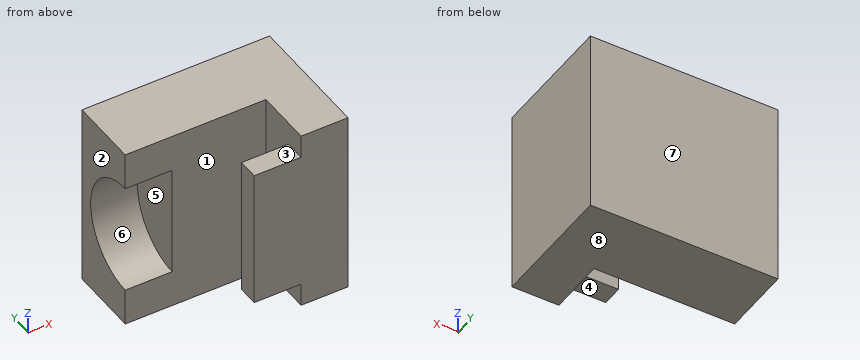
from build123d import *

# Parameters (mm, degrees)
SKETCH1_W           = 25.4
SKETCH1_H           = 9.525
BOSS_EXTRUDE1_DEPTH = 25.4
SKETCH2_W           = 6.35
SKETCH2_H           = 25.4
BOSS_EXTRUDE2_DEPTH = 7.747
SKETCH3_W           = 19.05
SKETCH3_H           = 2.794
BOSS_EXTRUDE3_DEPTH = 6.35
CUT_EXTRUDE1_DEPTH  = 6.35


with BuildPart() as part:
    # Sketch1 → Boss-Extrude1 (new body)
    with BuildSketch(Plane(origin=(0, 0, 0), x_dir=(0, 0, -1), z_dir=(1, 0, 0))):
        Rectangle(SKETCH1_W, SKETCH1_H)
    extrude(amount=BOSS_EXTRUDE1_DEPTH)

    # Sketch2 → Boss-Extrude2 (add)
    with BuildSketch(Plane.XZ.offset(4.7625)):
        with Locations((22.225, 0)):
            Rectangle(SKETCH2_W, SKETCH2_H)
    extrude(amount=BOSS_EXTRUDE2_DEPTH)

    # Sketch3 → Boss-Extrude3 (add)
    with BuildSketch(Plane.ZY.offset(-19.05)):
        with Locations((0, -11.1125)):
            Rectangle(SKETCH3_W, SKETCH3_H)
    extrude(amount=BOSS_EXTRUDE3_DEPTH)

    # Sketch4 → Cut-Extrude1 (cut)
    with BuildSketch(Plane.ZY):
        with BuildLine():
            Line((-7.62, -4.7625), (7.62, -4.7625))
            ThreePointArc((7.62, -4.7625), (0, 2.8575), (-7.62, -4.7625))
        make_face()
    extrude(amount=-CUT_EXTRUDE1_DEPTH, mode=Mode.SUBTRACT)


solid = part.part
The listing builds one solid part. Answer for the finished solid, in the listing's coordinates (mm). Face numbers are marked on the shaded views. A direction names the side the tool comes from. Coordinates: 2 decimals unless noted, no trailing zeros. Loops run counter-clockwise (first coordinate to the right, second up) from the corner with the lowest first, then second, coordinate; pieces in that order, holes last. Notation, with made-up numbers: (-9, -13) -> (18, -13) arc R35 cw to (18, 22) -> close; hole circle Ø10 at (26, 83.5). An arc over 180 degrees is marked (long way). Answer in a Markdown table with one row per item. Add a question column.
1. For the marked faces 1, 2, 3 and 4, determine the directions among +Z, -Z, +X, -X, +Y, -Y from which every point of the face is accessible in a straight line to the end or side of a thin tool.
2. Consider line 1 (Y direction, x = 17.5, z = -4.75); line 2 (X direction, y = -6, z = -4); line 3 (Y direction, x = 10.5, z = -8.5). Determine where each line is inside the solid, lowest interval first. Write a range as [from, to].
3. The part is cut by section C-C, the plane x = 8.5. Write down the section's boundary in (y, z), then the cut area to 3 significant figures.
4. The part is cut by section B-B, the plane y = 1.75. Write down the section's boundary in (x, z), then the cut area to 3 significant figures.
5. Determine the mould class of the marked faces 5, 6, 7 and 8 for opening direction Z: +Z half, -Z half, draft (parallel to the pull), parting line (faces both ways), or undercut.
6. The part is cut by section A-A, the plane z = 0. Write down the section's boundary in (x, y).
7. Flat-ended cylindrical pins translate along their axes: P1, Ø2, axis at x = 14.5, y = -11.5, coming from the +Z side (3 decimals); P2, Ø2, axis at y = -10.5, z = -3, coming from the -X side; P3, Ø2, axis at x = 12, z = -7.5, coming from the -Y side; P4, Ø3, axis at x = 17, y = -11.5, coming from the -Z side (3 decimals). Find the tip coordinate at first contact, or state that the pin passes through.
8. The part is cut by section D-D, the plane z = -5. Write down the section's boundary in (x, y).
Answer below:
| question | item | result |
|---|---|---|
| 1 | face 1 | +Z, -Z, -X |
| 1 | face 2 | +Z, -Z, -X, +Y, -Y |
| 1 | face 3 | +Z, -X, -Y |
| 1 | face 4 | -Z, -X, -Y |
| 2 | line 1 | [-12.51, -9.72], [-4.76, 4.76] |
| 2 | line 2 | [19.05, 25.4] |
| 2 | line 3 | [-4.76, 4.76] |
| 3 | outline | (-4.76, -12.7) -> (4.76, -12.7) -> (4.76, 12.7) -> (-4.76, 12.7) -> close |
| 3 | area | 242 mm2 |
| 4 | outline | (0, -12.7) -> (25.4, -12.7) -> (25.4, 12.7) -> (0, 12.7) -> (0, 3.96) -> (6.35, 3.96) -> (6.35, -3.96) -> (0, -3.96) -> close |
| 4 | area | 595 mm2 |
| 5 | face 5 | undercut |
| 5 | face 6 | undercut |
| 5 | face 7 | draft |
| 5 | face 8 | -Z half |
| 6 | outline | (0, 2.86) -> (6.35, 2.86) -> (6.35, -4.76) -> (19.05, -4.76) -> (19.05, -9.72) -> (12.7, -9.72) -> (12.7, -12.51) -> (25.4, -12.51) -> (25.4, 4.76) -> (0, 4.76) -> close |
| 7 | P1 | z = 9.525 |
| 7 | P2 | x = 12.7 |
| 7 | P3 | y = -12.51 |
| 7 | P4 | z = -9.525 |
| 8 | outline | (0, 0.99) -> (6.35, 0.99) -> (6.35, -4.76) -> (19.05, -4.76) -> (19.05, -9.72) -> (12.7, -9.72) -> (12.7, -12.51) -> (25.4, -12.51) -> (25.4, 4.76) -> (0, 4.76) -> close |
